from build123d import *

# Parameters (mm, degrees)
SKETCH_1_R          = 230
EXTRUDE_1_DEPTH     = 8
SKETCH_3_W          = 80
SKETCH_3_H          = 200
CUT_EXTRUDE_1_DEPTH = 10
SKETCH_4_R          = 3.75
SKETCH_4_R_2        = 2.75
CUT_EXTRUDE_2_DEPTH = 10
SKETCH_6_W          = 40
SKETCH_6_H          = 20
SKETCH_6_W_2        = 25
SKETCH_6_H_2        = 25
CUT_EXTRUDE_4_DEPTH = 10
FILLET_2_R          = 10
FILLET_3_R          = 10
FILLET_4_R          = 10
SKETCH_7_R          = 2.75
SKETCH_7_R_2        = 3.75
CUT_EXTRUDE_5_DEPTH = 10
SKETCH_8_R          = 1.5
CUT_EXTRUDE_6_DEPTH = 326.005785815
SKETCH_9_R          = 2.25
CUT_EXTRUDE_7_DEPTH = 11
FILLET_5_R          = 3
SKETCH_10_R         = 1.65
CUT_EXTRUDE_8_DEPTH = 10


with BuildPart() as part:
    # 草图1 → 凸台-拉伸1 (new body)
    with BuildSketch(Plane(origin=(0, 0, 0), x_dir=(0, 0, -1), z_dir=(1, 0, 0))):
        Circle(SKETCH_1_R)
    extrude(amount=EXTRUDE_1_DEPTH)

    # 草图3 → 切除-拉伸1 (cut)
    with BuildSketch(Plane(origin=(8, 0, 0), x_dir=(0, 0, -1), z_dir=(1, 0, 0))):
        with Locations((190, 95)):
            Rectangle(SKETCH_3_W, SKETCH_3_H)
        with Locations((-190, 95)):
            Rectangle(SKETCH_3_W, SKETCH_3_H)
    extrude(amount=-CUT_EXTRUDE_1_DEPTH, mode=Mode.SUBTRACT)

    # 草图4 → 切除-拉伸2 (cut)
    with BuildSketch(Plane(origin=(8, 0, 0), x_dir=(0, 0, -1), z_dir=(1, 0, 0))):
        with Locations((166.813442197, -81.229769803)):
            Circle(SKETCH_4_R)
        with Locations((108.962557326, -150.173769684)):
            Circle(SKETCH_4_R)
        with Locations((-108.962557326, -150.173769684)):
            Circle(SKETCH_4_R)
        with Locations((-166.813442197, -81.229769803)):
            Circle(SKETCH_4_R)
        with Locations((-45, 190)):
            Circle(SKETCH_4_R)
        with Locations((45, 190)):
            Circle(SKETCH_4_R)
        with Locations((-12.5, 35)):
            Circle(SKETCH_4_R_2)
        with Locations((12.5, 35)):
            Circle(SKETCH_4_R_2)
        with Locations((-50.5, 202.5)):
            Circle(SKETCH_4_R_2)
        with Locations((50.5, 202.5)):
            Circle(SKETCH_4_R_2)
        with Locations((-50.5, 177.5)):
            Circle(SKETCH_4_R_2)
        with Locations((50.5, 177.5)):
            Circle(SKETCH_4_R_2)
        with Locations((179.92432959, -85.051370487)):
            Circle(SKETCH_4_R_2)
        with Locations((115.002781011, -162.421859242)):
            Circle(SKETCH_4_R_2)
        with Locations((160.773218512, -68.981680245)):
            Circle(SKETCH_4_R_2)
        with Locations((95.851669933, -146.352169)):
            Circle(SKETCH_4_R_2)
        with Locations((-160.773218512, -68.981680245)):
            Circle(SKETCH_4_R_2)
        with Locations((-179.92432959, -85.051370487)):
            Circle(SKETCH_4_R_2)
        with Locations((-95.851669933, -146.352169)):
            Circle(SKETCH_4_R_2)
        with Locations((-115.002781011, -162.421859242)):
            Circle(SKETCH_4_R_2)
        with Locations((12.5, 136)):
            Circle(SKETCH_4_R_2)
        with Locations((-12.5, 136)):
            Circle(SKETCH_4_R_2)
        with Locations((0, 130.5)):
            Circle(SKETCH_4_R)
        with Locations((0, 40.5)):
            Circle(SKETCH_4_R)
    extrude(amount=-CUT_EXTRUDE_2_DEPTH, mode=Mode.SUBTRACT)

    # 草图6 → 切除-拉伸4 (cut)
    with BuildSketch(Plane(origin=(8, 0, 0), x_dir=(0, 0, -1), z_dir=(1, 0, 0))):
        with Locations((0, 160)):
            Rectangle(SKETCH_6_W, SKETCH_6_H)
        with Locations((-102.5, -92.5)):
            Rectangle(SKETCH_6_W_2, SKETCH_6_H_2)
        with Locations((102.5, -92.5)):
            Rectangle(SKETCH_6_W_2, SKETCH_6_H_2)
    extrude(amount=-CUT_EXTRUDE_4_DEPTH, mode=Mode.SUBTRACT)

    # 圆角2
    fillet_2_edges = [part.edges().sort_by_distance(p)[0] for p in [
        (4, -5, 229.945645751),
    ]]
    fillet(fillet_2_edges, radius=FILLET_2_R)

    # 圆角3
    fillet_3_edges = [part.edges().sort_by_distance(p)[0] for p in [
        (4, 174.355957742, -150),
        (4, -5, -229.945645751),
        (4, 174.355957742, 150),
    ]]
    fillet(fillet_3_edges, radius=FILLET_3_R)

    # 圆角4
    fillet_4_edges = [part.edges().sort_by_distance(p)[0] for p in [
        (4, -5, -150),
        (4, -5, 150),
    ]]
    fillet(fillet_4_edges, radius=FILLET_4_R)

    # 草图7 → 切除-拉伸5 (cut)
    with BuildSketch(Plane(origin=(8, 0, 0), x_dir=(0, 0, -1), z_dir=(1, 0, 0))):
        with Locations((85, 40)):
            Circle(SKETCH_7_R)
        with Locations((110, 40)):
            Circle(SKETCH_7_R)
        with Locations((85, -61)):
            Circle(SKETCH_7_R)
        with Locations((110, -61)):
            Circle(SKETCH_7_R)
        with Locations((97.5, 34.5)):
            Circle(SKETCH_7_R_2)
        with Locations((97.5, -55.5)):
            Circle(SKETCH_7_R_2)
        with Locations((-97.5, -55.5)):
            Circle(SKETCH_7_R_2)
        with Locations((-97.5, 34.5)):
            Circle(SKETCH_7_R_2)
        with Locations((-110, -61)):
            Circle(SKETCH_7_R)
        with Locations((-85, -61)):
            Circle(SKETCH_7_R)
        with Locations((-110, 40)):
            Circle(SKETCH_7_R)
        with Locations((-85, 40)):
            Circle(SKETCH_7_R)
    extrude(amount=-CUT_EXTRUDE_5_DEPTH, mode=Mode.SUBTRACT)

    # 草图8 → 切除-拉伸6 (cut, through all)
    with BuildSketch(Plane(origin=(8, 0, 0), x_dir=(0, 0, -1), z_dir=(1, 0, 0))):
        with Locations((-59, 169)):
            Circle(SKETCH_8_R)
        with Locations((-59, 90)):
            Circle(SKETCH_8_R)
        with Locations((59, 169)):
            Circle(SKETCH_8_R)
        with Locations((59, 90)):
            Circle(SKETCH_8_R)
    extrude(amount=-CUT_EXTRUDE_6_DEPTH, mode=Mode.SUBTRACT)

    # 草图9 → 切除-拉伸7 (cut)
    with BuildSketch(Plane(origin=(8, 0, 0), x_dir=(0, 0, -1), z_dir=(1, 0, 0))):
        with Locations((70, 4.25)):
            Circle(SKETCH_9_R)
        with Locations((70, -61.25)):
            Circle(SKETCH_9_R)
        with Locations((-70, 4.25)):
            Circle(SKETCH_9_R)
        with Locations((-70, -61.25)):
            Circle(SKETCH_9_R)
    extrude(amount=-CUT_EXTRUDE_7_DEPTH, mode=Mode.SUBTRACT)

    # 圆角5
    fillet_5_edges = [part.edges().sort_by_distance(p)[0] for p in [
        (4, -105, 115),
        (4, -80, 115),
        (4, -80, 90),
        (4, -105, 90),
        (4, 150, 20),
        (4, 170, 20),
        (4, 170, -20),
        (4, 150, -20),
        (4, -105, -90),
        (4, -80, -90),
        (4, -80, -115),
        (4, -105, -115),
    ]]
    fillet(fillet_5_edges, radius=FILLET_5_R)

    # 草图10 → 切除-拉伸8 (cut)
    with BuildSketch(Plane(origin=(8, 0, 0), x_dir=(0, 0, -1), z_dir=(1, 0, 0))):
        with Locations((-59, -85)):
            Circle(SKETCH_10_R)
        with Locations((59, -85)):
            Circle(SKETCH_10_R)
        with Locations((59, -164)):
            Circle(SKETCH_10_R)
        with Locations((-59, -164)):
            Circle(SKETCH_10_R)
    extrude(amount=-CUT_EXTRUDE_8_DEPTH, mode=Mode.SUBTRACT)


solid = part.part
Geometry: final body of the model. Coordinates: model frame, mm. Round coordinates to 2 decimals unless told otherwise and drop trailing zeros. Order: outer loops, then holes, each group sorted by start corner. A loop starts at its lowest first (then second) coordinate and runs counter-clockwise, first axis right, second up.
Q1. Pin query (flat end, axial travel): pin 1 (2.5 mm diameter, centred on x = 5, z = -99, fed in from +Y); pin 2 (3 mm diameter, centred on x = 7, y = -85.5, fed in from -Z); pin 3 (2.5 mm diameter, centred on x = 5, y = 126.5, fed in from -Z). Return the tip coordinate at first contact, or that it passes through.
Result sheet:
pin 1: stops at y = 208.19
pin 2: stops at z = -214.11
pin 3: stops at z = -150
Q2. Mould query, pull axis Y, two halves, no side actions, for faces 1 (the face through (3.94, -2.15, 153.01)), 2 (the face through (8, 3, 3)), 3 (the face through (3.94, -229.95, 4.84)). Classes: released by +Y, released by -Y, zero draft, split by the parting line, or undercut.
Result sheet:
face 1: released by +Y
face 2: zero draft
face 3: released by -Y
Q3. Material intervals for probe 1 along Y at (x, z) = (2.25, 11); probe 2 along Z at (x, y) = (4.75, 163.5); probe 3 along Y at (x, z) = (2, 97), sorted ascending.
Result sheet:
probe 1: y = -229.74 to 32.7, 37.3 to 133.7, 138.3 to 150, 170 to 229.74
probe 2: z = -150 to -20, 20 to 150
probe 3: y = -208.54 to -148.85, -143.85 to -105, -80 to -59.22, -51.78 to 30.78, 38.22 to 208.54
Q4. Section A-A, the plane y = 65. Output: boundary loops of the cut face in (x, z), and give its area (3 significant figures).
Result sheet:
outline: (0, -150) - (8, -150) - (8, 150) - (0, 150) - close
area: 2,400 mm2
Q5. Section B-B, the plane z = 124. Output: boundary loops of the cut face in (x, y), and give its area (3 significant figures).
Result sheet:
outline: (0, -193.71) - (8, -193.71) - (8, 193.71) - (0, 193.71) - close
area: 3,100 mm2
Q6. Section C-C, the plane x = 4.75. Give the number of separate pieces and of enclosed holes in the cut face, and give its area (3 significant figures).
Result sheet:
separate pieces: 1
enclosed holes: 51
area: 143,000 mm2
